Build history of the part. All positions in model axes, mm. A direction names the side the tool comes from. Give positions to 0.01 mm unless a question says otherwise; leave off trailing zeros. Loops run counter-clockwise (first coordinate to the right, second up) from the corner with the lowest first, then second, coordinate; pieces in that order, holes last. Notation, with made-up numbers: M 67,46 L 110,46 A33 cw 110,83 Z; hole C -29.75,13 d9. An arc over 180 degrees is marked long. Put each result on its own line as item: value.
```python
from build123d import *

# Parameters (mm, degrees)
F1_DEPTH = 10


with BuildPart() as f1:
    # F0 (on Top) → F1 (new body)
    with BuildSketch(Plane.XY):
        Polygon((0, -45), (65, -45), (65, -35), (75, -35), (75, -25), (65, -25), (65, -15), (75, -15), (75, -5), (65, -5), (65, 5), (75, 5), (75, 15), (65, 15), (65, 25), (-65, 25), (-65, 15), (-75, 15), (-75, 5), (-65, 5), (-65, -5), (-75, -5), (-75, -15), (-65, -15), (-65, -25), (-75, -25), (-75, -35), (-65, -35), (-65, -45), align=None)
    extrude(amount=F1_DEPTH)


solid = f1.part
```
Q1. Probe line 1 (X direction, y = 3, z = 5.5). List the from-to ranges inside material, lowest first. Write a range as from..to.
Here are the results:
line 1: -65..65
Q2. Drop flat-ended pins along their axis: pin 1 Ø3 at (x, z) = (-68.5, 5.5) entering from -Y; pin 2 Ø6 at (x, y) = (43, -11.5) entering from -Z; pin 3 Ø3 at (y, z) = (0.5, 4) entering from -X; pin 4 Ø3 at (x, z) = (70.5, 4.5) entering from +Y. Give the stop position or say it passes through.
Here are the results:
pin 1: y = -35
pin 2: z = 0
pin 3: x = -65
pin 4: y = 15
Q3. Mould opens along Y. For faces 1 (the flat face through (70, -35, 5)), 2 (the flat face through (75, -30, 5)), 3 (the flat face through (-65, 0, 5)) say: pulls with the +Y half, pulls with the -Y half, needs draft (parallel to the pull), parting line crosses it, or undercut.
Here are the results:
face 1: pulls with the -Y half
face 2: needs draft
face 3: undercut
Q4. Slice it at B-B (y = -19). List the corners of the cut face in (x, z), and give its area (3 significant figures).
Here are the results:
outline: M -65,0 L 65,0 L 65,10 L -65,10 Z
area: 1,300 mm²
Q5. Tool access for faces 4 (the flat face through (70, -25, 5)), 5 (the flat face through (-70, -25, 5)), 6 (the flat face through (65, -40, 5)), 7 (the flat face through (-65, -40, 5)): list every direction of +Z, -Z, +X, -X, +Y, -Y with a clear straight run to the whole face (end or side of a thin tool).
Here are the results:
face 4: +Z, -Z, +X
face 5: +Z, -Z, -X
face 6: +Z, -Z, +X, -Y
face 7: +Z, -Z, -X, -Y
Q6. Slice it at A-A (z = 1.75). List the corners of the cut face in (x, y), and give its area (3 significant figures).
Here are the results:
outline: M -75,-35 L -65,-35 L -65,-45 L 65,-45 L 65,-35 L 75,-35 L 75,-25 L 65,-25 L 65,-15 L 75,-15 L 75,-5 L 65,-5 L 65,5 L 75,5 L 75,15 L 65,15 L 65,25 L -65,25 L -65,15 L -75,15 L -75,5 L -65,5 L -65,-5 L -75,-5 L -75,-15 L -65,-15 L -65,-25 L -75,-25 Z
area: 9,700 mm²
